```python
from build123d import *

# Parameters (mm, degrees)
F1_DEPTH = 101.6
F2_DEPTH = 50.8
F3_R     = 25.4
F4_DEPTH = 101.6


with BuildPart() as f1:
    # F0 (on Front) → F1 (new body)
    with BuildSketch(Plane.XZ):
        Polygon((30.294443, 168.60885), (-20.505557, 168.60885), (-20.505557, 16.20885), (81.094443, 16.20885), (81.094443, 168.60885), align=None)
    extrude(amount=F1_DEPTH)

    # F0 (on Front) → F2 (join)
    with BuildSketch(Plane.XZ):
        with BuildLine():
            Line((30.294443, 244.80885), (-20.505557, 168.60885))
            Line((-20.505557, 168.60885), (30.294443, 168.60885))
            Line((30.294443, 168.60885), (30.294443, 194.00885))
            ThreePointArc((30.294443, 194.00885), (17.594443, 206.70885), (30.294443, 219.40885))
            Line((30.294443, 219.40885), (30.294443, 244.80885))
        make_face()
        Polygon((30.294443, 168.60885), (-20.505557, 168.60885), (-20.505557, 16.20885), (81.094443, 16.20885), (81.094443, 168.60885), align=None)
        with BuildLine():
            Line((30.294443, 194.00885), (30.294443, 168.60885))
            Line((30.294443, 168.60885), (81.094443, 168.60885))
            Line((81.094443, 168.60885), (30.294443, 244.80885))
            Line((30.294443, 244.80885), (30.294443, 219.40885))
            ThreePointArc((30.294443, 219.40885), (39.274699, 215.689107), (42.994443, 206.70885))
            ThreePointArc((42.994443, 206.70885), (39.274699, 197.728594), (30.294443, 194.00885))
        make_face()
    extrude(amount=F2_DEPTH)

    # F3 (on face) → F4 (join)
    with BuildSketch(Plane(origin=(0, 0, 16.20885), x_dir=(1, 0, 0), z_dir=(0, 0, -1))):
        with Locations((30.294443, 50.8)):
            Circle(F3_R)
    extrude(amount=F4_DEPTH)


solid = f1.part
```
Check sheet for the modelled part. Datum: model origin and axes. Units: mm. A direction names the side the tool comes from. Coordinates: 2 decimals unless noted, no trailing zeros. Loops run counter-clockwise (first coordinate to the right, second up) from the corner with the lowest first, then second, coordinate; pieces in that order, holes last. Notation, with made-up numbers: M 9,66.5 L 24,66.5 A23 cw 24,98.5 Z; hole C 63.25,68.25 d6. An arc over 180 degrees is marked long. Answer as a JSON object with one key per item and string values.
1. Scan lines: L1, parallel to Z at x = 30.5, y = -84.5; L2, parallel to X at y = -38.5, z = 203.5; L3, parallel to Z at x = 19, y = -41. Record each from-to range of solid material in increasing order. Write a range as from..to.
Outcome:
{"L1": "16.21..168.61", "L2": "2.76..18.01, 42.58..57.83", "L3": "-85.39..200.9, 212.52..227.87"}
2. Sectioned sample at B-B on x = 65. Record the cut outline in (y, z).
Outcome:
{"outline": "M -101.6,16.21 L 0,16.21 L 0,192.75 L -50.8,192.75 L -50.8,168.61 L -101.6,168.61 Z"}
3. Sectioned sample at C-C on y = -72. Record the cut outline in (x, z), and give its area (3 significant figures).
Outcome:
{"outline": "M -20.51,16.21 L 16.3,16.21 L 16.3,-85.39 L 44.28,-85.39 L 44.28,16.21 L 81.09,16.21 L 81.09,168.61 L -20.51,168.61 Z", "area": "18,300 mm²"}
4. Sectioned sample at A-A on y = -22. Record the cut outline in (x, z).
Outcome:
{"outline": "M -20.51,16.21 L 81.09,16.21 L 81.09,168.61 L 30.29,244.81 L -20.51,168.61 Z; hole M 30.29,219.41 A12.7 ccw long 42.99,206.71 A12.7 ccw Z"}
5. Sectioned sample at D-D on z = -47. Record the cut outline in (x, y).
Outcome:
{"outline": "C 30.29,-50.8 d50.8"}
6. Release check for a two-part mould opening along X. For faces 4 (the flat face through (81.094, -50, 91)), 5 (the flat face through (-20.506, -50, 93)), 6 (the flat face through (30, -50.8, 190)) record: pulls with the +X half, pulls with the -X half, needs draft (parallel to the pull), parting line crosses it, or undercut.
Outcome:
{"face 4": "pulls with the +X half", "face 5": "pulls with the -X half", "face 6": "needs draft"}
7. Depth check by flat-ended pin: P1, Ø12, axis at x = 59, z = 5.5, coming from the +Y side (3 decimals); P2, Ø2, axis at x = 14, y = -29.5, coming from the +Z side; P3, Ø8, axis at x = 50.5, y = -10.5, coming from the -Z side. Enter the tip coordinate at first touch or a pass-through.
Outcome:
{"P1": "y = -39.415", "P2": "z = 221.87", "P3": "z = 16.21"}
8. Access from +Z, -Z, +X, -X, +Y, -Y to the whole of each face (thin tool, end or side, straight path). Record for faces 1 (the flat face through (7, -39, 16.209)), 2 (the flat face through (31, -76, 168.609)), 3 (the flat face through (5.25, -25.04, 207.24)).
Outcome:
{"face 1": "-Z", "face 2": "+Z, +X, -X, -Y", "face 3": "+Z, -X, +Y, -Y"}
